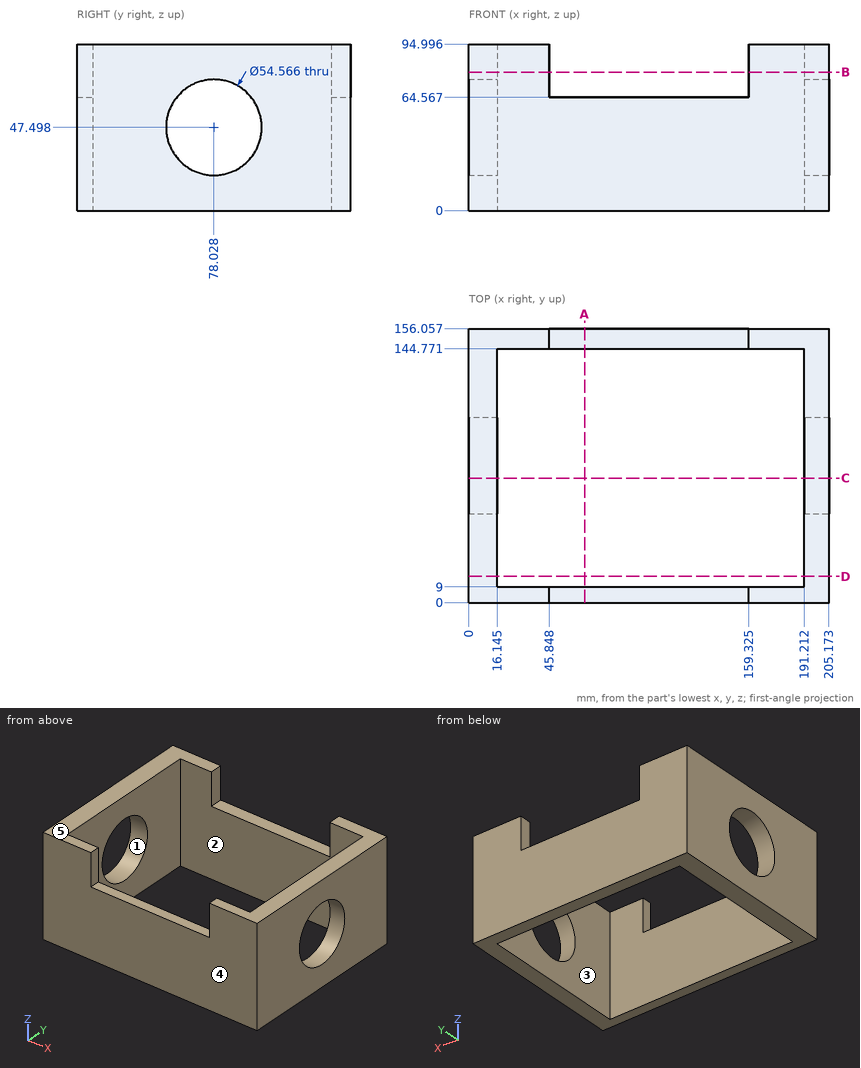
Drawing for the job (mm, zero at the part's lowest x, y, z). A direction names the side the tool comes from. Give positions to 0.01 mm unless a question says otherwise; leave off trailing zeros. Loops run counter-clockwise (first coordinate to the right, second up) from the corner with the lowest first, then second, coordinate; pieces in that order, holes last.
Item 1: Slice it at B-B (z = 79). Write the cut outline in (x, y) (1 decimal), plus the area to 3 significant figures.
Check values:
outline: (0, 0) - (45.8, 0) - (45.8, 9) - (16.1, 9) - (16.1, 144.8) - (45.8, 144.8) - (45.8, 156.1) - (0, 156.1) - close; (159.3, 0) - (205.2, 0) - (205.2, 156.1) - (159.3, 156.1) - (159.3, 144.8) - (191.2, 144.8) - (191.2, 9) - (159.3, 9) - close
area: 5,950 mm2
Item 2: Drill centre lines: line 1 along X through (y, z) = (141, 88) (1 decimal); line 2 along Y through (x, z) = (18.5, 60); line 3 along Z through (x, y) = (194.5, 72.5) (1 decimal). Where is each one in solid material? Low to high.
Check values:
line 1: x = 0 to 16.1, 191.2 to 205.2
line 2: y = 0 to 9, 144.77 to 156.06
line 3: z = 0 to 20.8, 74.2 to 95
Item 3: Slice it at C-C (y = 71). Write the cut outline in (x, z) (1 decimal), plus the area to 3 significant figures.
Check values:
outline: (0, 0) - (16.1, 0) - (16.1, 21.1) - (0, 21.1) - close; (0, 73.9) - (16.1, 73.9) - (16.1, 95) - (0, 95) - close; (191.2, 0) - (205.2, 0) - (205.2, 21.1) - (191.2, 21.1) - close; (191.2, 73.9) - (205.2, 73.9) - (205.2, 95) - (191.2, 95) - close
area: 1,270 mm2
Item 4: Mould opens along Y. For the marked faces 3, 4 and 5 say: +Y half, -Y half, draft (parallel to the pull), parting line (faces both ways), or undercut.
Check values:
face 3: undercut
face 4: -Y half
face 5: draft
Item 5: Slice it at D-D (y = 15). Write the cut outline in (x, z) (1 decimal).
Check values:
outline: (0, 0) - (16.1, 0) - (16.1, 95) - (0, 95) - close; (191.2, 0) - (205.2, 0) - (205.2, 95) - (191.2, 95) - close
Item 6: Drop a flat-ended pin along its axis: P1, Ø7, axis at x = 116, y = 5.5, coming from the +Z side. Give the stop position or say it passes through.
Check values:
P1: stops at z = 64.57
Item 7: Slice it at A-A (x = 66). Write the cut outline in (y, z), plus the area to 3 significant figures.
Check values:
outline: (0, 0) - (9, 0) - (9, 64.57) - (0, 64.57) - close; (144.77, 0) - (156.06, 0) - (156.06, 64.57) - (144.77, 64.57) - close
area: 1,310 mm2
Item 8: Which spindle directions (+Z, -Z, +X, -X, +Y, -Y) get a long thin tool onto all of the face, cutting with end or side? Do the marked faces 1 and 2. Say none if no direction does.
Check values:
face 1: +X, -X
face 2: +Z, -Z
